Could you check a few things on this model? Use its own coordinates, in mm. Face numbers are marked on the shaded views. Give positions to 0.01 mm unless a question says otherwise; leave off trailing zeros. Loops run counter-clockwise (first coordinate to the right, second up) from the corner with the lowest first, then second, coordinate; pieces in that order, holes last. Notation, with made-up numbers: (-32, -30) - (22, -30) arc R31 ccw to (22, -1) - close; hole circle Ø7 at (49, 27.25). An arc over 180 degrees is marked (long way). Write each question's results on one line, items separated by ' | '. Start each with the question number.
(1) Suppose I cut it at D-D (x = 0.5). Please give me the cut outline in (y, z).
(2) If we mould it in two halves opening along Y, with no side actions, what happens to the marked faces 1 and 2? For each: released by +Y, released by -Y, zero draft, split by the parting line, or undercut.
(3) Suppose I cut it at C-C (y = 13). Please give me the cut outline in (x, z), and give its area (3 significant figures).
(4) Suppose I cut it at A-A (z = -27.5). Please give me the cut outline in (x, y) (3 decimals), and give its area (3 significant figures).
(5) Suppose I cut it at B-B (x = 29.5). Please give me the cut outline in (y, z) (3 decimals).
(6) For pin 1 (1.9 mm diameter, centred on x = 34.5, z = -30.5, fed in from -Y) (3 decimals); pin 2 (3 mm diameter, centred on x = 23.5, y = -12.5, fed in from +Z); pin 3 (1.1 mm diameter, centred on y = 31, z = -26, fed in from -X); pin 4 (7 mm diameter, centred on x = 34, z = -30, fed in from +Y), each with a flat end and sliding along its axis, tell me the tip position at first contact or that it passes through.
(7) I need wall thicknesses on line 1 (Z direction, x = 56, y = -16.5); line 2 (X direction, y = -30, z = -30.5). Which ranges of each line are inside material? Lowest first, please.
from build123d import *

# Parameters (mm, degrees)
SKETCH005_W  = 128.778
SKETCH005_H  = 67.818
PAD004_DEPTH = 2.9972
SKETCH006_W  = 10.16
SKETCH006_H  = 2.54
PAD005_DEPTH = 10.16
SKETCH007_R  = 1.905
PAD006_DEPTH = 10.16
SKETCH008_R  = 1.905
PAD007_DEPTH = 10.16


with BuildPart() as part:
    # Sketch005 → Pad004 (new body)
    with BuildSketch(Plane(origin=(0, 0, -32.258), x_dir=(1, 0, 0), z_dir=(0, 0, -1))):
        Rectangle(SKETCH005_W, SKETCH005_H)
    extrude(amount=PAD004_DEPTH)

    # Sketch006 → Pad005 (new body)
    with BuildSketch(Plane.XY.offset(-32.258)):
        with Locations((-33.02, -29.845)):
            Rectangle(SKETCH006_W, SKETCH006_H)
        with Locations((33.02, -29.845)):
            Rectangle(SKETCH006_W, SKETCH006_H)
        with Locations((33.02, 29.845)):
            Rectangle(SKETCH006_W, SKETCH006_H)
        with Locations((-33.02, 29.845)):
            Rectangle(SKETCH006_W, SKETCH006_H)
    extrude(amount=PAD005_DEPTH)

    # Sketch007 → Pad006 (new body)
    with BuildSketch(Plane(origin=(38.1, 0, -32.258), x_dir=(0, -1, 0), z_dir=(1, 0, 0))):
        with Locations((-30.48, -8.255)):
            Circle(SKETCH007_R)
        with Locations((30.48, -8.255)):
            Circle(SKETCH007_R)
    extrude(amount=-PAD006_DEPTH)

    # Sketch008 → Pad007 (new body)
    with BuildSketch(Plane(origin=(-38.1, 0, -32.258), x_dir=(0, 1, 0), z_dir=(-1, 0, 0))):
        with Locations((-30.48, -8.255)):
            Circle(SKETCH008_R)
        with Locations((30.48, -8.255)):
            Circle(SKETCH008_R)
    extrude(amount=-PAD007_DEPTH)


solid = part.part
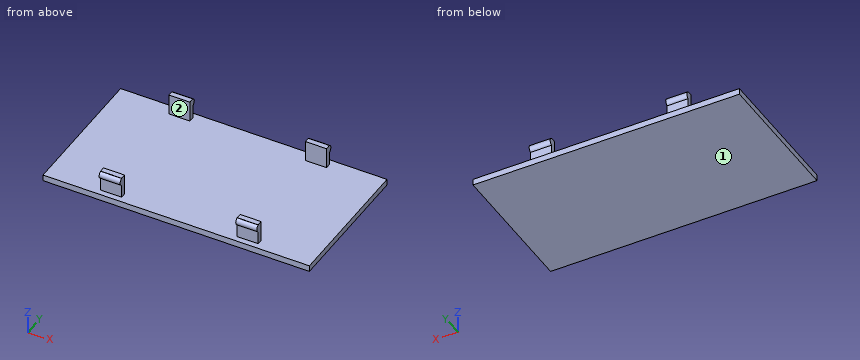
Output values:
1) outline: (-33.91, -35.26) - (33.91, -35.26) - (33.91, -32.26) - (-33.91, -32.26) - close
2) face 1: zero draft | face 2: undercut
3) outline: (-64.39, -35.26) - (64.39, -35.26) - (64.39, -32.26) - (-64.39, -32.26) - close | area: 386 mm2
4) outline: (-38.1, -31.115) - (-27.94, -31.115) - (-27.94, -28.575) - (-38.1, -28.575) - close; (-38.1, 28.575) - (-27.94, 28.575) - (-27.94, 31.115) - (-38.1, 31.115) - close; (27.94, -31.115) - (38.1, -31.115) - (38.1, -28.575) - (27.94, -28.575) - close; (27.94, 28.575) - (38.1, 28.575) - (38.1, 31.115) - (27.94, 31.115) - close | area: 103 mm2
5) outline: (-33.909, -35.255) - (33.909, -35.255) - (33.909, -32.258) - (31.115, -32.258) - (31.115, -25.799) arc R1.905 ccw to (31.115, -22.207) - (31.115, -22.098) - (28.575, -22.098) - (28.575, -32.258) - (-28.575, -32.258) - (-28.575, -22.098) - (-31.115, -22.098) - (-31.115, -22.207) arc R1.905 ccw to (-31.115, -25.799) - (-31.115, -32.258) - (-33.909, -32.258) - close
6) pin 1: y = -31.115 | pin 2: z = -32.26 | pin 3: x = -38.1 | pin 4: y = 33.91
7) line 1: -35.26 to -32.26 | line 2: -38.1 to -27.94, 27.94 to 38.1
